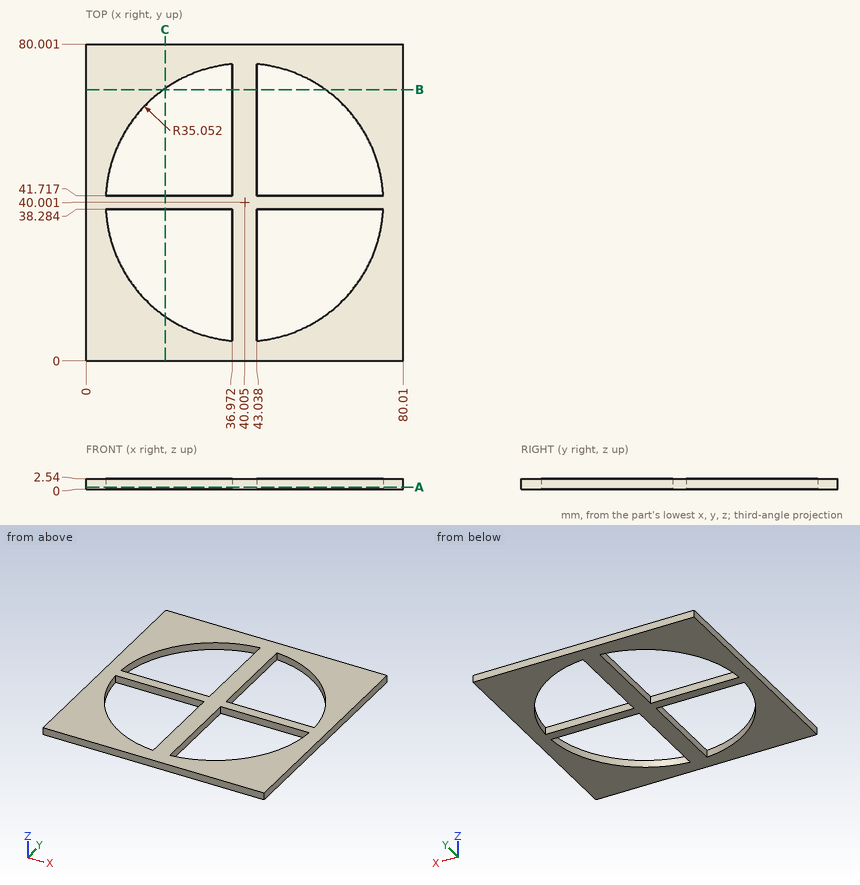
Study the drawing (mm; zero at the part's minimum x, y, z) and answer. Round coordinates to 2 decimals unless told otherwise and drop trailing zeros. Loops run counter-clockwise (first coordinate to the right, second up) from the corner with the lowest first, then second, coordinate; pieces in that order, holes last. Notation, with made-up numbers: (20.25, 51) -> (61.25, 51) arc R7 ccw to (61.25, 58) -> close; hole circle Ø10 at (63, 29). An arc over 180 degrees is marked (long way). Write each question's results on one line, items separated by ' | '. Start each with the question number.
1. Given pin 1 Ø0.8 at (x, z) = (66.5, 1) entering from -Y; pin 2 Ø5 at (x, y) = (26.5, 45.5) entering from +Z, each flat-ended and moving along its own axis, determine where each tip first touches the part or whether it passes through.
2. Section C-C (x = 20) is taken. Determine the outline of the cut face in (y, z).
3. Find the intervals of material crossed by probe 1 along X at (y, z) = (42, 0.25); probe 2 along X at (y, z) = (60.5, 0.25); probe 3 along Y at (x, z) = (45.5, 1.4) (1 decimal), in increasing order. Write a range as from..to.
4. Section A-A (z = 0.5) is taken. Determine the outline of the cut face in (x, y) (1 decimal).
5. Section B-B (y = 68.5) is taken. Determine the outline of the cut face in (x, z).
Evaluation:
1) pin 1: stops at y = 0 | pin 2: passes through
2) outline: (0, 0) -> (11.22, 0) -> (11.22, 2.54) -> (0, 2.54) -> close; (38.28, 0) -> (41.72, 0) -> (41.72, 2.54) -> (38.28, 2.54) -> close; (68.78, 0) -> (80, 0) -> (80, 2.54) -> (68.78, 2.54) -> close
3) probe 1: x = 0..5.01, 36.97..43.04, 75..80.01 | probe 2: x = 0..11.57, 36.97..43.04, 68.44..80.01 | probe 3: y = 0..5.4, 38.3..41.7, 74.6..80
4) outline: (0, 0) -> (80, 0) -> (80, 80) -> (0, 80) -> close; hole (5, 38.3) arc R35.1 ccw to (37, 5.1) -> (37, 38.3) -> close; hole (5, 41.7) -> (37, 41.7) -> (37, 74.9) arc R35.1 ccw to start; hole (43, 5.1) arc R35.1 ccw to (75, 38.3) -> (43, 38.3) -> close; hole (43, 41.7) -> (75, 41.7) arc R35.1 ccw to (43, 74.9) -> close
5) outline: (0, 0) -> (19.6, 0) -> (19.6, 2.54) -> (0, 2.54) -> close; (36.97, 0) -> (43.04, 0) -> (43.04, 2.54) -> (36.97, 2.54) -> close; (60.41, 0) -> (80.01, 0) -> (80.01, 2.54) -> (60.41, 2.54) -> close
